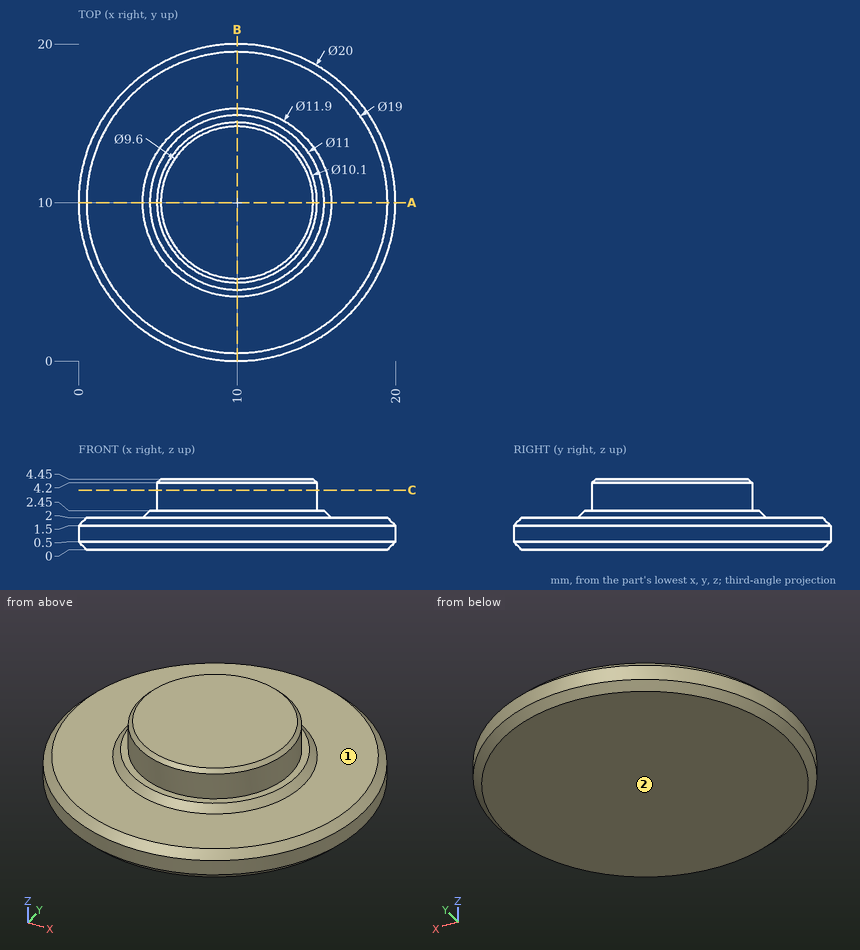
The drawing under review shows one solid part. Ordinate dimensions are in mm from its lowest x, y, z. A direction names the side the tool comes from. Give positions to 0.01 mm unless a question says otherwise; leave off trailing zeros. Write each loop counter-clockwise with the first axis right and the second up, starting at its lowest first coordinate (ties: lowest second). Pieces come first, ordered by that corner, then holes. Notation, with made-up numbers: M 16,-33.5 L 49,-33.5 A19 ccw 49,-17.5 Z; hole C 57,-16.75 d7. An arc over 180 degrees is marked long. Write each question's results on one line, items separated by ' | '. Start each with the question number.
1. We need section A-A (y = 10). Write out the cut boundary in (x, z), and give its area (3 significant figures).
2. For the marked faces 1 and 2, list the 3-axis set-ups (+Z, -Z, +X, -X, +Y, -Y) from which the entire face can be reached by the end or side of a thin tool; tool diameter is ignored.
3. We need section C-C (z = 3.75). Write out the cut boundary in (x, y).
4. For probe 1 along Z at (x, y) = (12.25, 18); probe 2 along Y at (x, z) = (12, 0.25); probe 3 along Z at (x, y) = (3, 16.5), list the stretches that pass through material, from the lowest coordinate up. Write a range as [from, to].
5. Insertion check: pin 1 Ø5 at (x, y) = (2, 16) entering from +Z. The pin has a flat end and moves straight along its axis. Give the tip position at first contact, or say it passes through.
Results found:
1) outline: M 0,0.5 L 0.5,0 L 19.5,0 L 20,0.5 L 20,1.5 L 19.5,2 L 15.95,2 L 15.5,2.45 L 15.05,2.45 L 15.05,4.2 L 14.8,4.45 L 5.2,4.45 L 4.95,4.2 L 4.95,2.45 L 4.5,2.45 L 4.05,2 L 0.5,2 L 0,1.5 Z | area: 64.8 mm^2
2) face 1: +Z | face 2: -Z, +X, -X, +Y, -Y
3) outline: C 10,10 d10.1
4) probe 1: z = [0, 2] | probe 2: y = [0.46, 19.54] | probe 3: z = [0.05, 1.95]
5) pin 1: stops at z = 2
